from build123d import *

# Parameters (mm, degrees)
F0_W     = 101.614196
F0_H     = 86.362857
F1_DEPTH = 50.8
F2_R     = 25.4
F3_R     = 25.4


with BuildPart() as f1:
    # F0 (on Right) → F1 (new body)
    with BuildSketch(Plane.YZ):
        with Locations((-1.026405, 0.513206)):
            Rectangle(F0_W, F0_H)
    extrude(amount=F1_DEPTH)

    # F2
    f2_edges = [f1.edges().sort_by_distance(p)[0] for p in [
        (25.4, -51.833503, 43.694634),
    ]]
    fillet(f2_edges, radius=F2_R)

    # F3
    f3_edges = [f1.edges().sort_by_distance(p)[0] for p in [
        (25.4, 49.780693, 43.694634),
        (25.4, -51.833503, -42.668223),
        (25.4, 49.780693, -42.668223),
    ]]
    fillet(f3_edges, radius=F3_R)


solid = f1.part
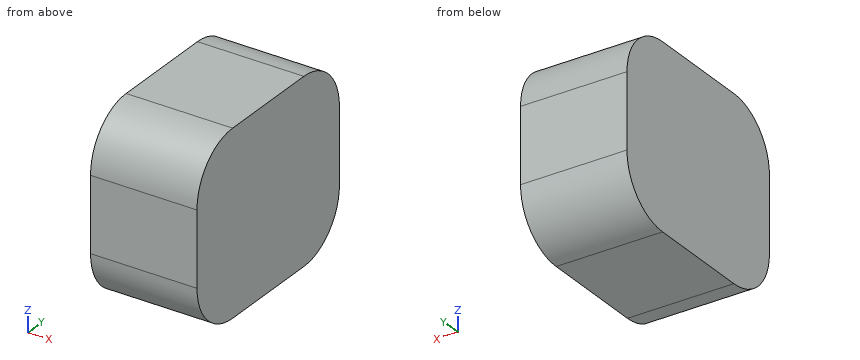
Model file for the job. Use its own axes, mm. Give positions to 0.01 mm unless a question says otherwise; leave off trailing zeros. Loops run counter-clockwise (first coordinate to the right, second up) from the corner with the lowest first, then second, coordinate; pieces in that order, holes last.
Item 1: Drop flat-ended pins along their axis: P1, Ø3, axis at x = 32, z = 25, coming from the +Y side; P2, Ø6, axis at x = 5.5, z = -26.5, coming from the +Y side; P3, Ø1.5, axis at x = 11.5, y = -37, coming from the -Z side. Give the stop position or say it passes through.
Check values:
P1: stops at y = 49.24
P2: stops at y = 49
P3: stops at z = -40.69
Item 2: Slice it at A-A (x = 22). Write the cut outline in (y, z).
Check values:
outline: (-51.83, -17.27) arc R25.4 ccw to (-26.43, -42.67) - (24.38, -42.67) arc R25.4 ccw to (49.78, -17.27) - (49.78, 18.29) arc R25.4 ccw to (24.38, 43.69) - (-26.43, 43.69) arc R25.4 ccw to (-51.83, 18.29) - close
Item 3: Slice it at B-B (y = 35). Write the cut outline in (x, z), plus the area to 3 significant figures.
Check values:
outline: (0, -40.34) - (50.8, -40.34) - (50.8, 41.37) - (0, 41.37) - close
area: 4,150 mm2
Item 4: Slice it at C-C (z = 36). Write the cut outline in (x, y).
Check values:
outline: (0, -44.65) - (50.8, -44.65) - (50.8, 42.59) - (0, 42.59) - close
Item 5: Drill centre lines: line 1 along Z through (x, y) = (28, 25.5); line 2 along Z through (x, y) = (23, -27); line 3 along Y through (x, z) = (19.5, 28). Where is each one in solid material? Low to high.
Check values:
line 1: z = -42.64 to 43.67
line 2: z = -42.66 to 43.69
line 3: y = -49.91 to 47.85
